Read the model definition and answer for the solid it produces. Units are mm, in the model's axes. A direction names the side the tool comes from. Give positions to 0.01 mm unless a question says otherwise; leave off trailing zeros. Loops run counter-clockwise (first coordinate to the right, second up) from the corner with the lowest first, then second, coordinate; pieces in that order, holes last. Notation, with made-up numbers: (89.25, 25) -> (135.25, 25) arc R28 cw to (135.25, 63) -> close; hole circle Ø5 at (-38, 73.25). An arc over 180 degrees is marked (long way). Answer as CSV lines item,"result". Start each with the question number.
```python
from build123d import *

# Parameters (mm, degrees)
F1_DEPTH = 59.944
F0_R     = 9.5854875755
F2_DEPTH = 34.544


with BuildPart() as f1:
    # F0 (on Top) → F1 (new body)
    with BuildSketch(Plane.XY):
        Polygon((42.7391566336, -44.3220846355), (-42.4513481557, -13.3829666302), (-42.4513481557, -44.3220846355), align=None)
    extrude(amount=F1_DEPTH)

    # F0 (on Top) → F2 (join)
    with BuildSketch(Plane.XY):
        with BuildLine():
            ThreePointArc((42.7391566336, 15.8293172717), (0.9256115544, 55.2569720027), (-42.4513481557, 17.5561513752))
            Line((-42.4513481557, 17.5561513752), (-42.4513481557, -13.3829666302))
            Line((-42.4513481557, -13.3829666302), (42.7391566336, -44.3220846355))
            Line((42.7391566336, -44.3220846355), (42.7391566336, 15.8293172717))
        make_face()
        Circle(F0_R, mode=Mode.SUBTRACT)
    extrude(amount=F2_DEPTH)


solid = f1.part
```
(1) Find the intervals of material crossed by line 1 along Y through (x, z) = (0, 12.5); line 2 along Z through (x, y) = (-5.5, 26); line 3 along Y through (x, z) = (-1.5, 11), in increasing order. Write a range as from..to.
(2) Find section A-A on x = 1. Write down the section's boundary in (y, z).
(3) Each of these flat-tipped pins is pushed along its axis until it touches: P1, Ø3, axis at y = 23.5, z = 9, coming from the +X side; P2, Ø8, axis at x = 25, z = 19, coming from the +Y side. Where does it stop, or does it pass through?
(4) Find section B-B on y = -2. Write down the section's boundary in (x, z).
(5) Find section C-C on z = 14. Write down the section's boundary in (x, y).
(6) The mould has two halves that part along X. Classify faces 3 (the face through (-7.61, -5.83, 17.03)), 4 (the face through (1.81, 55.23, 17.03)), 5 (the face through (0.74, -29.07, 47.07)): pulls with the +X half, pulls with the -X half, needs draft (parallel to the pull), parting line crosses it, or undercut.
(7) A tool of negligible diameter and unlimited length cuts with its end or side. For faces 1 (the face through (-19, -36, 59.944)), 2 (the face through (9, 6, 34.544)), from which of +Z, -Z, +X, -X, +Y, -Y can it reach the whole face along a straight path? Write none if from no direction.
(8) Find section D-D on x = 24. Write down the section's boundary in (y, z).
Answer block:
1,line 1,"y = -44.32..-9.59, 9.59..55.27"
1,line 2,"z = 0..34.54"
1,line 3,"y = -44.32..-9.47, 9.47..55.24"
2,outline,"(-44.32, 0) -> (-9.53, 0) -> (-9.53, 34.54) -> (-29.16, 34.54) -> (-29.16, 59.94) -> (-44.32, 59.94) -> close; (9.53, 0) -> (55.26, 0) -> (55.26, 34.54) -> (9.53, 34.54) -> close"
3,P1,"stops at x = 41.79"
3,P2,"stops at y = 49.79"
4,outline,"(-42.45, 0) -> (-9.37, 0) -> (-9.37, 34.54) -> (-42.45, 34.54) -> close; (9.37, 0) -> (42.74, 0) -> (42.74, 34.54) -> (9.37, 34.54) -> close"
5,outline,"(-42.45, -44.32) -> (42.74, -44.32) -> (42.74, 15.83) arc R42.81 ccw to (-42.45, 17.56) -> close; hole circle Ø19.17 at (0, 0)"
6,face 3,"undercut"
6,face 4,"parting line crosses it"
6,face 5,"pulls with the +X half"
7,face 1,"+Z, +X, -X, +Y, -Y"
7,face 2,"+Z, +X, +Y"
8,outline,"(-44.32, 0) -> (47.95, 0) -> (47.95, 34.54) -> (-37.52, 34.54) -> (-37.52, 59.94) -> (-44.32, 59.94) -> close"
